from build123d import *

# Parameters (mm, degrees)
BOSS_EXTRUDE1_DEPTH            = 1.0000005
BOSS_EXTRUDE1_DEPTH_BACK       = 3
SKETCH1_R                      = 7.4
SKETCH1_R_2                    = 6.5
BOSS_EXTRUDE2_DEPTH            = 1.0000005
BOSS_EXTRUDE12_START           = -3
BOSS_EXTRUDE12_DEPTH           = 4.000001
SKETCH6_W                      = 2.880295876
SKETCH6_H                      = 10.5
BOSS_EXTRUDE8_DEPTH            = 0.5
CIRPATTERN3_COUNT              = 4
SKETCH7_R                      = 14
SKETCH7_R_2                    = 10
BOSS_EXTRUDE10_DEPTH           = 1.0000005
M2_CLEARANCE_HOLE1_D           = 2.4
M2_CLEARANCE_HOLE1_CSINK_D     = 2.45
M2_CLEARANCE_HOLE1_CSINK_ANGLE = 90
CUT_EXTRUDE1_DEPTH             = 28.738141627


with BuildPart() as part:
    # Sketch1 → Boss-Extrude1 (new, two sides: drawn at the far end of the back side and taken through both)
    with BuildSketch(Plane.XY.offset(-BOSS_EXTRUDE1_DEPTH_BACK)):
        Circle(SKETCH1_R)
        Circle(SKETCH1_R_2, mode=Mode.SUBTRACT)
    extrude(amount=BOSS_EXTRUDE1_DEPTH + BOSS_EXTRUDE1_DEPTH_BACK)

    # Sketch2 → Boss-Extrude2 (add)
    with BuildSketch(Plane.XY.offset(1.0000005)):
        with BuildLine():
            ThreePointArc((2.0955, -15.598818832), (6.979767945, -14.106633498), (11.129112031, -11.129112031))
            ThreePointArc((11.129112031, -11.129112031), (14.106633498, -6.979767945), (15.598818832, -2.0955))
            Line((15.598818832, -2.0955), (19.408818832, -2.0955))
            Line((19.408818832, -2.0955), (19.408818832, 2.0955))
            Line((19.408818832, 2.0955), (15.598818832, 2.0955))
            ThreePointArc((15.598818832, 2.0955), (11.129112031, 11.129112031), (2.0955, 15.598818832))
            Line((2.0955, 15.598818832), (2.0955, 19.408818832))
            Line((2.0955, 19.408818832), (-2.0955, 19.408818832))
            Line((-2.0955, 19.408818832), (-2.0955, 15.598818832))
            ThreePointArc((-2.0955, 15.598818832), (-11.129112031, 11.129112031), (-15.598818832, 2.0955))
            Line((-15.598818832, 2.0955), (-19.408818832, 2.0955))
            Line((-19.408818832, 2.0955), (-19.408818832, -2.0955))
            Line((-19.408818832, -2.0955), (-15.598818832, -2.0955))
            ThreePointArc((-15.598818832, -2.0955), (-11.129112031, -11.129112031), (-2.0955, -15.598818832))
            Line((-2.0955, -15.598818832), (-2.0955, -19.408818832))
            Line((-2.0955, -19.408818832), (2.0955, -19.408818832))
            Line((2.0955, -19.408818832), (2.0955, -15.598818832))
        make_face()
        with BuildLine():
            ThreePointArc((7.4, 0), (7.323884446, -1.05863904), (7.097103617, -2.0955))
            Line((7.097103617, -2.0955), (13.031535896, -2.0955))
            ThreePointArc((13.031535896, -2.0955), (11.753270525, -6.006053615), (9.333060807, -9.333060807))
            ThreePointArc((9.333060807, -9.333060807), (6.006053615, -11.753270525), (2.0955, -13.031535896))
            Line((2.0955, -13.031535896), (2.0955, -7.097103617))
            ThreePointArc((2.0955, -7.097103617), (0, -7.4), (-2.0955, -7.097103617))
            Line((-2.0955, -7.097103617), (-2.0955, -13.031535896))
            ThreePointArc((-2.0955, -13.031535896), (-9.333060807, -9.333060807), (-13.031535896, -2.0955))
            Line((-13.031535896, -2.0955), (-7.097103617, -2.0955))
            ThreePointArc((-7.097103617, -2.0955), (-7.4, 0), (-7.097103617, 2.0955))
            Line((-7.097103617, 2.0955), (-13.031535896, 2.0955))
            ThreePointArc((-13.031535896, 2.0955), (-9.333060807, 9.333060807), (-2.0955, 13.031535896))
            Line((-2.0955, 13.031535896), (-2.0955, 7.097103617))
            ThreePointArc((-2.0955, 7.097103617), (0, 7.4), (2.0955, 7.097103617))
            Line((2.0955, 7.097103617), (2.0955, 13.031535896))
            ThreePointArc((2.0955, 13.031535896), (9.333060807, 9.333060807), (13.031535896, 2.0955))
            Line((13.031535896, 2.0955), (7.097103617, 2.0955))
            ThreePointArc((7.097103617, 2.0955), (7.323884446, 1.05863904), (7.4, 0))
        make_face(mode=Mode.SUBTRACT)
    extrude(amount=-BOSS_EXTRUDE2_DEPTH)

    # Sketch3 → Boss-Extrude12 (add)
    with BuildSketch(Plane.XY.offset(BOSS_EXTRUDE12_START)):
        with BuildLine():
            ThreePointArc((4.867078755, 5.574185536), (4.880275394, 5.562635354), (4.893444623, 5.551053929))
            ThreePointArc((4.893444623, 5.551053929), (5.244976244, 5.220174729), (5.574185536, 4.867078755))
            Line((5.574185536, 4.867078755), (6.858935778, 6.151828996))
            Line((6.858935778, 6.151828996), (6.151828996, 6.858935778))
            Line((6.151828996, 6.858935778), (4.867078755, 5.574185536))
        make_face()
        with BuildLine():
            ThreePointArc((-4.893444623, 5.551053929), (-4.880275394, 5.562635354), (-4.867078755, 5.574185536))
            Line((-4.867078755, 5.574185536), (-6.151828996, 6.858935778))
            Line((-6.151828996, 6.858935778), (-6.858935778, 6.151828996))
            Line((-6.858935778, 6.151828996), (-5.574185536, 4.867078755))
            ThreePointArc((-5.574185536, 4.867078755), (-5.244976244, 5.220174729), (-4.893444623, 5.551053929))
        make_face()
        with BuildLine():
            Line((6.858935778, -6.151828996), (5.574185536, -4.867078755))
            ThreePointArc((5.574185536, -4.867078755), (5.232590181, -5.232590181), (4.867078755, -5.574185536))
            Line((4.867078755, -5.574185536), (6.151828996, -6.858935778))
            Line((6.151828996, -6.858935778), (6.858935778, -6.151828996))
        make_face()
        with BuildLine():
            ThreePointArc((-4.867078755, -5.574185536), (-5.232590181, -5.232590181), (-5.574185536, -4.867078755))
            Line((-5.574185536, -4.867078755), (-6.858935778, -6.151828996))
            Line((-6.858935778, -6.151828996), (-6.151828996, -6.858935778))
            Line((-6.151828996, -6.858935778), (-4.867078755, -5.574185536))
        make_face()
    extrude(amount=BOSS_EXTRUDE12_DEPTH)

    # Sketch6 → Boss-Extrude8 (add)
    with BuildSketch(Plane(origin=(0, 0, 0), x_dir=(-1, 0, 0), z_dir=(0, 0, -1))):
        with Locations((0.009852062, 14.158818832)):
            Rectangle(SKETCH6_W, SKETCH6_H)
    boss_extrude8 = extrude(amount=BOSS_EXTRUDE8_DEPTH)

    # CirPattern3: Boss-Extrude8 ×4 about axis
    cirpattern3_axis = Axis((0, 0, 0), (0, 0, 1))
    for i in range(1, CIRPATTERN3_COUNT):
        add(boss_extrude8.rotate(cirpattern3_axis, i * 360 / CIRPATTERN3_COUNT))

    # Sketch7 → Boss-Extrude10 (add)
    with BuildSketch(Plane.XY.offset(1.0000005)):
        Circle(SKETCH7_R)
        Circle(SKETCH7_R_2, mode=Mode.SUBTRACT)
    extrude(amount=-BOSS_EXTRUDE10_DEPTH)

    # M2 Clearance Hole1 (through all)
    with Locations(Plane.XY.offset(1.0000005)):
        with Locations((0, 0), (8.485, -8.485), (-8.485, 8.485), (-8.485, -8.485), (8.485, 8.485)):
            CounterSinkHole(M2_CLEARANCE_HOLE1_D / 2, M2_CLEARANCE_HOLE1_CSINK_D / 2, counter_sink_angle=M2_CLEARANCE_HOLE1_CSINK_ANGLE)

    # Sketch10 → Cut-Extrude1 (cut, through all)
    with BuildSketch(Plane.XY.offset(1.0000005)):
        with BuildLine():
            ThreePointArc((-2.0955, 13.83682648), (-9.895678028, 9.895678028), (-13.83682648, 2.0955))
            Line((-13.83682648, 2.0955), (-20.600743229, 2.0955))
            ThreePointArc((-20.600743229, 2.0955), (-14.335944494, 14.286228168), (-2.0955, 20.453324327))
            Line((-2.0955, 20.453324327), (-2.0955, 13.83682648))
        make_face()
        with BuildLine():
            ThreePointArc((13.83682648, 2.0955), (9.895678028, 9.895678028), (2.0955, 13.83682648))
            Line((2.0955, 13.83682648), (2.0955, 20.453324327))
            ThreePointArc((2.0955, 20.453324327), (15.477172624, 15.2424301), (21.254785436, 2.0955))
            Line((21.254785436, 2.0955), (13.83682648, 2.0955))
        make_face()
        with BuildLine():
            ThreePointArc((-2.0955, -21.163548472), (-15.297243757, -15.462085596), (-20.600743229, -2.0955))
            Line((-20.600743229, -2.0955), (-13.83682648, -2.0955))
            ThreePointArc((-13.83682648, -2.0955), (-9.895678028, -9.895678028), (-2.0955, -13.83682648))
            Line((-2.0955, -13.83682648), (-2.0955, -21.163548472))
        make_face()
        with BuildLine():
            ThreePointArc((2.0955, -13.83682648), (9.895678028, -9.895678028), (13.83682648, -2.0955))
            Line((13.83682648, -2.0955), (21.254785436, -2.0955))
            ThreePointArc((21.254785436, -2.0955), (15.624264861, -15.597542172), (2.0955, -21.163548472))
            Line((2.0955, -21.163548472), (2.0955, -13.83682648))
        make_face()
    extrude(amount=-CUT_EXTRUDE1_DEPTH, mode=Mode.SUBTRACT)


solid = part.part
Can you work these out from the model? Positions are in its coordinate system, mm. A direction names the side the tool comes from. Give positions to 0.01 mm unless a question says otherwise; leave off trailing zeros. Loops run counter-clockwise (first coordinate to the right, second up) from the corner with the lowest first, then second, coordinate; pieces in that order, holes last. Notation, with made-up numbers: (37, 33) -> (95, 33) arc R33 ccw to (95, 70) -> close; hole circle Ø7 at (63, 43.25). An arc over 180 degrees is marked (long way). Use one line per item in the form item = value.
1) For faces 1 (the face through (14, 0, -0.5)), 2 (the face through (-14, 0, -0.5)), 3 (the face through (6.208, 5.5, -1.028)), which set-ups out of +Z, -Z, +X, -X, +Y, -Y let a thin tool reach every point of the face, with its end or its side?
Answers:
face_1 = -Z, +X, +Y, -Y
face_2 = -Z, -X, +Y, -Y
face_3 = +Z, -Z
2) If we section it at A-A (x = 0): Please give me the cut outline in (y, z), plus the area to 3 significant figures.
Answers:
outline = (-19.41, -0.5) -> (-8.91, -0.5) -> (-8.91, 0) -> (-7.4, 0) -> (-7.4, -3) -> (-6.5, -3) -> (-6.5, 1) -> (-19.41, 1) -> close; (6.5, -3) -> (7.4, -3) -> (7.4, 0) -> (8.91, 0) -> (8.91, -0.5) -> (19.41, -0.5) -> (19.41, 1) -> (6.5, 1) -> close
area = 41.7 mm²
3) If we section it at C-C (z = -2): Please give me the cut outline in (x, y), plus the area to 3 significant figures.
Answers:
outline = (-6.86, -6.15) -> (-6.15, -6.86) -> (-4.87, -5.57) arc R7.4 ccw to (4.87, -5.57) -> (6.15, -6.86) -> (6.86, -6.15) -> (5.57, -4.87) arc R7.4 ccw to (5.57, 4.87) -> (6.86, 6.15) -> (6.15, 6.86) -> (4.87, 5.57) arc R7.4 ccw to (-4.87, 5.57) -> (-6.15, 6.86) -> (-6.86, 6.15) -> (-5.57, 4.87) arc R7.4 ccw to (-5.57, -4.87) -> close; hole circle Ø13 at (0, 0)
area = 46.5 mm²
4) I need wall thicknesses on line 1 along X through (y, z) = (5.5, 0.65); line 2 along Y through (x, z) = (-1, -0.15); line 3 along Y through (x, z) = (14, -0.3). Which ranges of each line are inside material? Lowest first, please.
Answers:
line_1 = -12.87 to -8.35, -6.21 to -3.46, 3.46 to 6.21, 8.35 to 12.87
line_2 = -19.41 to -8.91, -7.33 to -6.42, 6.42 to 7.33, 8.91 to 19.41
line_3 = -1.43 to 1.45
5) If we section it at D-D (x = 14.5): Please give me the cut outline in (y, z).
Answers:
outline = (-2.1, 0) -> (-1.43, 0) -> (-1.43, -0.5) -> (1.45, -0.5) -> (1.45, 0) -> (2.1, 0) -> (2.1, 1) -> (-2.1, 1) -> close
6) Will these pins go through, and if not, where does the flat tip stop? pin 1 (1.1 mm diameter, centred on y = 16, z = 0.5, fed in from +X); pin 2 (0.9 mm diameter, centred on x = -12.5, y = 0.5, fed in from -Z); pin 3 (0.5 mm diameter, centred on y = 17.5, z = 0.5, fed in from -X).
Answers:
pin_1 = 2.1
pin_2 = -0.5
pin_3 = -2.1
